from build123d import *

# Parameters (mm, degrees)
BOSS_EXTRUDE1_DEPTH = 10
SKETCH2_W           = 39
SKETCH2_H           = 2
BOSS_EXTRUDE2_DEPTH = 10


with BuildPart() as part:
    # Sketch1 → Boss-Extrude1 (new body)
    with BuildSketch(Plane.XY):
        with BuildLine():
            Line((-19.5, 20), (-19.5, 0))
            Line((-19.5, 0), (-17.5, 0))
            Line((-17.5, 0), (-17.5, 8))
            ThreePointArc((-17.5, 8), (-14.571067812, 15.071067812), (-7.5, 18))
            Line((-7.5, 18), (7.5, 18))
            ThreePointArc((7.5, 18), (14.571067812, 15.071067812), (17.5, 8))
            Line((17.5, 8), (17.5, 0))
            Line((17.5, 0), (19.5, 0))
            Line((19.5, 0), (19.5, 20))
            Line((19.5, 20), (-19.5, 20))
        make_face()
    extrude(amount=BOSS_EXTRUDE1_DEPTH)

    # Sketch2 → Boss-Extrude2 (add)
    with BuildSketch(Plane.XY.offset(10)):
        with Locations((0, 19)):
            Rectangle(SKETCH2_W, SKETCH2_H)
    extrude(amount=BOSS_EXTRUDE2_DEPTH)


solid = part.part
Verification items for the finished model (mm, model axes). A direction names the side the tool comes from. Coordinates: 2 decimals unless noted, no trailing zeros. Order: outer loops, then holes, each group sorted by start corner. A loop starts at its lowest first (then second) coordinate and runs counter-clockwise, first axis right, second up. Notation, with made-up numbers: M 72,69 L 130,69 A29 ccw 130,99 Z; hole C 83.25,18.25 d2. An arc over 180 degrees is marked long. One line per item, written item: value. Start each with the question number.
Item 1: Sectioned sample at D-D on y = 17.5. Record the cut outline in (x, z).
Item 2: Sectioned sample at A-A on y = 6. Record the cut outline in (x, z), then the cut area to 3 significant figures.
Item 3: Sectioned sample at B-B on z = 6.25. Record the cut outline in (x, y), then the cut area to 3 significant figures.
Item 4: Thickness scan on probe 1 along X at (y, z) = (5, 2); probe 2 along Y at (x, z) = (7, 16); probe 3 along X at (y, z) = (15.5, 5). Record the ranges inside material, lowest first.
Item 5: Sectioned sample at C-C on x = -3. Record the cut outline in (y, z), then the cut area to 3 significant figures.
Item 6: Depth check by flat-ended pin: P1, Ø1.5, axis at x = 5, y = 16, coming from the -Z side; P2, Ø3, axis at x = -9, z = 14.5, coming from the -Y side; P3, Ø10, axis at x = -4.5, z = 10.5, coming from the -Y side. Enter the tip coordinate at first touch or a pass-through.
Item 7: Access from +Z, -Z, +X, -X, +Y, -Y to the whole of each face (thin tool, end or side, straight path). Record for faces 1 (the flat face through (-17.5, 4, 5)), 2 (the flat face through (17, 12, 10)), 3 (the flat face through (0, 20, 10)), 4 (the flat face through (0, 18, 12)).
Item 8: Mould release check, pull along X, two halves, no side actions. Record for faces 5 (the flat face through (19.5, 10, 5)), 6 (the flat face through (-19.5, 10, 5)), 7 (the flat face through (18, 0, 5)), 8 (the cylindrical face through (14.49, 15.15, 4.93)): pulls with the +X half, pulls with the -X half, needs draft (parallel to the pull), parting line crosses it, or undercut.
Calculated:
1. outline: M -19.5,0 L -10.62,0 L -10.62,10 L -19.5,10 Z; M 10.62,0 L 19.5,0 L 19.5,10 L 10.62,10 Z
2. outline: M -19.5,0 L -17.5,0 L -17.5,10 L -19.5,10 Z; M 17.5,0 L 19.5,0 L 19.5,10 L 17.5,10 Z
2. area: 40.0 mm^2
3. outline: M -19.5,0 L -17.5,0 L -17.5,8 A10 cw -7.5,18 L 7.5,18 A10 cw 17.5,8 L 17.5,0 L 19.5,0 L 19.5,20 L -19.5,20 Z
3. area: 193 mm^2
4. probe 1: -19.5 to -17.5, 17.5 to 19.5
4. probe 2: 18 to 20
4. probe 3: -19.5 to -14.11, 14.11 to 19.5
5. outline: M 18,0 L 20,0 L 20,20 L 18,20 Z
5. area: 40.0 mm^2
6. P1: through
6. P2: y = 18
6. P3: y = 17.8
7. face 1: +Z, -Z, -Y
7. face 2: +Z, +X, -X, -Y
7. face 3: +Z, -Z, +X, -X, +Y
7. face 4: +Z, -Y
8. face 5: pulls with the +X half
8. face 6: pulls with the -X half
8. face 7: needs draft
8. face 8: undercut
